```python
from build123d import *

# Parameters (mm, degrees)
SKETCH1_R           = 8.5
BOSS_EXTRUDE1_DEPTH = 14.06
SKETCH4_R           = 6.355
CUT_EXTRUDE5_DEPTH  = 17.81
SKETCH5_R           = 1.59
CUT_EXTRUDE6_DEPTH  = 10


with BuildPart() as part:
    # Sketch1 → Boss-Extrude1 (new body)
    with BuildSketch(Plane(origin=(0, 0, 0), x_dir=(1, 0, 0), z_dir=(0, 1, 0))):
        with Locations(Location((0, 0, 0), (0, 0, 270))):
            Circle(SKETCH1_R)
    extrude(amount=BOSS_EXTRUDE1_DEPTH)

    # Loft1: read off the stored shape, not the designer's step
    # Loft1: loft between two sections, ruled curve by curve
    loft1_from = [
        Edge.make_bspline([(-1.303322944, 21.16, 6.214808871), (-13.732940686, 21.16, 3.608162984), (-11.126294799, 21.16, -8.821454758), (1.303322944, 21.16, -6.214808871), (13.732940686, 21.16, -3.608162984), (11.126294799, 21.16, 8.821454758), (-1.303322944, 21.16, 6.214808871)], [0, 0, 0, 0, 0.5, 0.5, 0.5, 1, 1, 1, 1], 3, [1, 0.333333333, 0.333333333, 1, 0.333333333, 0.333333333, 1]),
    ]
    loft1_to = [
        Edge.make_bspline([(1.802060434, 14.06, 8.30677905), (-14.811497666, 14.06, 11.910899919), (-18.415618535, 14.06, -4.702658182), (-1.802060434, 14.06, -8.30677905), (14.811497666, 14.06, -11.910899919), (18.415618535, 14.06, 4.702658182), (1.802060434, 14.06, 8.30677905)], [0, 0, 0, 0, 0.5, 0.5, 0.5, 1, 1, 1, 1], 3, [1, 0.333333333, 0.333333333, 1, 0.333333333, 0.333333333, 1]),
    ]
    loft1 = Solid(Shell([*[Face.make_surface_from_curves(loft1_from[k], loft1_to[k]) for k in range(1)], Face(Wire(loft1_from)), Face(Wire(loft1_to))]))
    add(loft1)

    # Sketch4 → Cut-Extrude5 (cut)
    with BuildSketch(Plane.XZ):
        with Locations(Location((0, 0, 0), (0, 0, 270))):
            Circle(SKETCH4_R)
    extrude(amount=-CUT_EXTRUDE5_DEPTH, mode=Mode.SUBTRACT)

    # Sketch5 → Cut-Extrude6 (cut, symmetric)
    with BuildSketch(Plane.XY):
        with Locations((0, 10.076564013)):
            Circle(SKETCH5_R)
        with Locations((0, 3.977190907)):
            Circle(SKETCH5_R)
    extrude(amount=CUT_EXTRUDE6_DEPTH, both=True, mode=Mode.SUBTRACT)


solid = part.part
```
CAD build for the part. Positions are in the model's coordinates, mm. A direction names the side the tool comes from. Round coordinates to 2 decimals unless told otherwise and drop trailing zeros. Write each loop counter-clockwise with the first axis right and the second up, starting at its lowest first coordinate (ties: lowest second). Pieces come first, ordered by that corner, then holes.
Item 1: Band-saw the part on A-A on y = 4.75. Write the cut outline in (x, z) (3 decimals).
Filled in:
outline: (-1.39, -8.386) - (-1.39, -6.201) arc R6.355 cw to (-1.39, 6.201) - (-1.39, 8.386) arc R8.5 ccw to start; (1.39, -8.386) arc R8.5 ccw to (1.39, 8.386) - (1.39, 6.201) arc R6.355 cw to (1.39, -6.201) - close
Item 2: Drop flat-ended pins along their axis: pin 1 Ø6 at (y, z) = (3, -6.5) entering from -X; pin 2 Ø4 at (x, y) = (6.5, 4.5) entering from -Z; pin 3 Ø1.9 at (x, y) = (0, 10.08) entering from -Z; pin 4 Ø5 at (x, z) = (0, -2.5) entering from -Y. Give the stop position or say it passes through.
Filled in:
pin 1: stops at x = -7.75
pin 2: stops at z = -7.21
pin 3: passes through
pin 4: stops at y = 17.81
Item 3: Tool access for faces 1 (the flat face through (-6, 0, 3)), 2 (the flat face through (0, 17.81, 0)): list every direction of +Z, -Z, +X, -X, +Y, -Y with a clear straight run to the whole face (end or side of a thin tool).
Filled in:
face 1: +Z, -Z, +X, -X, -Y
face 2: -Y
Item 4: Mould opens along X. For faces 3 (the cylindrical face through (1.5, 10.6, 7.3)), 4 (the flat face through (-1, 21.16, 0)), 5 (the cylindrical face through (-2.43, 8.78, -5.87)), 6 (the cylindrical face through (2.55, 6.93, 8.11)) say: released by +X, released by -X, zero draft, split by the parting line, or undercut.
Filled in:
face 3: undercut
face 4: zero draft
face 5: undercut
face 6: split by the parting line
Item 5: Drill centre lines: L1, parallel to X at y = 13.25, z = 0 (3 decimals); L2, parallel to Y at x = 3, z = -5.5; L3, parallel to X at y = 12, z = 4.25. Where is each one in solid material? Low to high.
Filled in:
L1: x = -8.5 to -6.355, 6.355 to 8.5
L2: y = 17.81 to 21.16
L3: x = -7.36 to -4.72, 4.72 to 7.36
Item 6: Band-saw the part on B-B on y = 7. Write the cut outline in (x, z) (3 decimals).
Filled in:
outline: circle Ø17 at (0, 0); hole circle Ø12.71 at (0, 0)
Item 7: Band-saw the part on C-C on x = 0. Give the number of separate pieces and of enclosed holes in the cut face, then the cut area to 3 significant figures.
Filled in:
separate pieces: 5
enclosed holes: 0
area: 89.3 mm2
